Work out the finished part from the listing and answer in its coordinate system (mm). A direction names the side the tool comes from. Coordinates: 2 decimals unless noted, no trailing zeros. Loops run counter-clockwise (first coordinate to the right, second up) from the corner with the lowest first, then second, coordinate; pieces in that order, holes last. Notation, with made-up numbers: (38, 87.5) -> (51, 87.5) arc R38 cw to (51, 125.5) -> close; hole circle Ø5 at (10.5, -37). An arc over 180 degrees is marked (long way). Use a Markdown table: item, result.
from build123d import *

# Parameters (mm, degrees)
SKETCH_1_W          = 24.7
SKETCH_1_H          = 24.7
SKETCH_1_W_2        = 12.7
SKETCH_1_H_2        = 12.7
EXTRUDE_2_DEPTH     = 24.7
EXTRUDE_3_DEPTH     = 14
EXTRUDE_5_DEPTH     = 14
SKETCH_6_R          = 2.5
CUT_EXTRUDE_1_DEPTH = 39.169817919
SKETCH_7_R          = 2.5
CUT_EXTRUDE_2_DEPTH = 44.755028282


with BuildPart() as part:
    # 草图1 → 凸台-拉伸2 (new body)
    # profile 1 of 2: a face of its own
    with BuildSketch(Plane(origin=(0, 0, 0), x_dir=(1, 0, 0), z_dir=(0, 1, 0))):
        Rectangle(SKETCH_1_W, SKETCH_1_H)
        Rectangle(SKETCH_1_W_2, SKETCH_1_H_2, mode=Mode.SUBTRACT)
    # profile 2 of 2: a face of its own
    with BuildSketch(Plane(origin=(0, 0, 0), x_dir=(1, 0, 0), z_dir=(0, 1, 0))):
        Rectangle(SKETCH_1_W_2, SKETCH_1_H_2)
    extrude(amount=EXTRUDE_2_DEPTH)

    # 草图3 → 凸台-拉伸3 (add)
    with BuildSketch(Plane.XZ):
        Polygon((-6.35, -6.35), (-6.35, 6.35), (-12.35, 6.35), (-12.35, -12.35), (12.35, -12.35), (12.35, 6.35), (6.35, 6.35), (6.35, -6.35), align=None)
    extrude(amount=EXTRUDE_3_DEPTH)

    # 草图5 → 凸台-拉伸5 (add)
    with BuildSketch(Plane(origin=(0, 0, -12.35), x_dir=(-1, 0, 0), z_dir=(0, 0, -1))):
        Polygon((6.35, 24.7), (-12.35, 24.7), (-12.35, 0), (6.35, 0), (6.35, 6), (-6.35, 6), (-6.35, 18.7), (6.35, 18.7), align=None)
    extrude(amount=EXTRUDE_5_DEPTH)

    # 草图6 → 切除-拉伸1 (cut, through all)
    with BuildSketch(Plane.XZ):
        with Locations(Location((0, -19.98, 0), (0, 0, 270))):
            Circle(SKETCH_6_R)
    extrude(amount=-CUT_EXTRUDE_1_DEPTH, mode=Mode.SUBTRACT)

    # 草图7 → 切除-拉伸2 (cut, through all)
    with BuildSketch(Plane.ZY.offset(12.35)):
        with Locations((0, -7.63)):
            Circle(SKETCH_7_R)
    extrude(amount=-CUT_EXTRUDE_2_DEPTH, mode=Mode.SUBTRACT)


solid = part.part
Q1. Given pin 1 Ø8 at (x, z) = (4.5, -17) entering from -Y; pin 2 Ø10 at (x, z) = (-9, -13.5) entering from -Y; pin 3 Ø5 at (y, z) = (4, -20) entering from -X; pin 4 Ø4.5 at (x, z) = (0, -19.98) entering from +Y, each flat-ended and moving along its own axis, determine where each tip first touches the part or whether it passes through.
Solved:
| item | result |
|---|---|
| pin 1 | y = 0 |
| pin 2 | y = -14 |
| pin 3 | x = -6.35 |
| pin 4 | through |
Q2. Section B-B on y = 0.5 is taken. Determine the outline of the cut face in (x, z), and give its area (3 significant figures).
Solved:
| item | result |
|---|---|
| outline | (-12.35, -12.35) -> (-6.35, -12.35) -> (-6.35, -26.35) -> (12.35, -26.35) -> (12.35, 12.35) -> (-12.35, 12.35) -> close; hole circle Ø5 at (0, -19.98) |
| area | 852 mm² |
Q3. For faces 1 (the flat face through (0, -7, -6.35)), 2 (the flat face through (-6.35, 22, -19)), 3 (the flat face through (3, 0, -19)), 4 (the flat face through (2, 18.7, -18)), 5 (the flat face through (-9, -7, 6.35)), determine the directions among +Z, -Z, +X, -X, +Y, -Y from which every point of the face is accessible in a straight line to the end or side of a thin tool.
Solved:
| item | result |
|---|---|
| face 1 | +Z, -Y |
| face 2 | -Z, -X, +Y, -Y |
| face 3 | -Z, +X, -X, -Y |
| face 4 | -Z, -X |
| face 5 | +Z, +X, -X, -Y |
Q4. Section A-A on x = -2 is taken. Determine the outline of the cut face in (y, z).
Solved:
| item | result |
|---|---|
| outline | (-14, -12.35) -> (0, -12.35) -> (0, -18.48) -> (6, -18.48) -> (6, -12.35) -> (18.7, -12.35) -> (18.7, -18.48) -> (24.7, -18.48) -> (24.7, 12.35) -> (0, 12.35) -> (0, -6.35) -> (-14, -6.35) -> close; (0, -26.35) -> (6, -26.35) -> (6, -21.48) -> (0, -21.48) -> close; (18.7, -26.35) -> (24.7, -26.35) -> (24.7, -21.48) -> (18.7, -21.48) -> close |
Q5. Section D-D on y = -7.63 is taken. Determine the outline of the cut face in (x, z), and give its area (3 significant figures).
Solved:
| item | result |
|---|---|
| outline | (-12.35, -12.35) -> (12.35, -12.35) -> (12.35, -2.5) -> (6.35, -2.5) -> (6.35, -6.35) -> (-6.35, -6.35) -> (-6.35, -2.5) -> (-12.35, -2.5) -> close; (-12.35, 2.5) -> (-6.35, 2.5) -> (-6.35, 6.35) -> (-12.35, 6.35) -> close; (6.35, 2.5) -> (12.35, 2.5) -> (12.35, 6.35) -> (6.35, 6.35) -> close |
| area | 241 mm² |
Q6. Section C-C on z = -19.98 is taken. Determine the outline of the cut face in (x, y).
Solved:
| item | result |
|---|---|
| outline | (-6.35, 0) -> (-2.5, 0) -> (-2.5, 6) -> (-6.35, 6) -> close; (-6.35, 18.7) -> (-2.5, 18.7) -> (-2.5, 24.7) -> (-6.35, 24.7) -> close; (2.5, 0) -> (12.35, 0) -> (12.35, 24.7) -> (2.5, 24.7) -> (2.5, 18.7) -> (6.35, 18.7) -> (6.35, 6) -> (2.5, 6) -> close |
Q7. Consider line 1 (X direction, y = 21.2, z = -19.98); line 2 (Y direction, x = -8, z = 0); line 3 (X direction, y = -3.5, z = 5.5). Determine where each line is inside the solid, lowest interval first. Write a range as [from, to].
Solved:
| item | result |
|---|---|
| line 1 | [-6.35, -2.5], [2.5, 12.35] |
| line 2 | [-14, -10.13], [-5.13, 24.7] |
| line 3 | [-12.35, -6.35], [6.35, 12.35] |
Q8. Determine the mould class of faces 6 (the flat face through (9, -7, 6.35)), 7 (the cylindrical face through (-9.39, -10.07, -0.54)), 8 (the cylindrical face through (0.11, 21.658, -17.482)), 9 (the flat face through (0, -14, -7)) for opening direction Z: pulls with the +Z half, pulls with the -Z half, needs draft (parallel to the pull), parting line crosses it, or undercut.
Solved:
| item | result |
|---|---|
| face 6 | pulls with the +Z half |
| face 7 | undercut |
| face 8 | undercut |
| face 9 | needs draft |
